Source: CAD feature listing. Evaluate the final solid. Frame: model axes, mm. A direction names the side the tool comes from. Coordinates: 2 decimals unless noted, no trailing zeros. Loops run counter-clockwise (first coordinate to the right, second up) from the corner with the lowest first, then second, coordinate; pieces in that order, holes last. Notation, with made-up numbers: (24.25, 89.25) - (70.25, 89.25) arc R26 cw to (70.25, 104.25) - close; hole circle Ø1 at (-14, -7). An arc over 180 degrees is marked (long way). Use one line per item in the form item = value. Start each with the question number.
from build123d import *

# Parameters (mm, degrees)
SKETCH1_R           = 15.175
SKETCH1_R_2         = 12
BOSS_EXTRUDE1_DEPTH = 20
BOSS_EXTRUDE2_REACH = 57.175
SKETCH2_R           = 12.675
SKETCH2_R_2         = 9.5
SKETCH5_W           = 2.65
SKETCH5_H           = 15.175


with BuildPart() as part:
    # Sketch1 → Boss-Extrude1 (new body, symmetric)
    with BuildSketch(Plane.XY):
        Circle(SKETCH1_R)
        Circle(SKETCH1_R_2, mode=Mode.SUBTRACT)
    extrude(amount=BOSS_EXTRUDE1_DEPTH, both=True)

    # Sketch2 → Boss-Extrude2 (add, up to next)
    with BuildSketch(Plane(origin=(0, 40, 0), x_dir=(1, 0, 0), z_dir=(0, 1, 0)), mode=Mode.PRIVATE) as boss_extrude2_sk1:
        Circle(SKETCH2_R)
        Circle(SKETCH2_R_2, mode=Mode.SUBTRACT)
    boss_extrude2_tool1 = extrude(boss_extrude2_sk1.sketch, amount=-BOSS_EXTRUDE2_REACH, mode=Mode.PRIVATE) - part.part
    add(boss_extrude2_tool1.solids().sort_by_distance((-12.316497, 40, 0))[0])

    # Sketch5 → M5 Clearance Hole1 (revolve, cut)
    with BuildSketch(Plane.ZX.offset(25.5)):
        with Locations((1.325, 7.5875)):
            Rectangle(SKETCH5_W, SKETCH5_H)
    m5_clearance_hole1 = revolve(axis=Axis((-6.35, 25.5, 0), (1, 0, 0)), mode=Mode.SUBTRACT)

    # Mirror1: M5 Clearance Hole1 across plane
    add(m5_clearance_hole1.mirror(Plane(origin=(0, 0, 0), x_dir=(0, 0, 1), z_dir=(1, 0, 0))), mode=Mode.SUBTRACT)


solid = part.part
(1) Mould query, pull axis X, two halves, no side actions, for faces 3 (the face through (-10.923, 23.709, -1.953)), 4 (the face through (12.09, 24.39, -3.81)), 5 (the face through (-11.99, 0.53, -0.28)). Classes: +X half, -X half, draft (parallel to the pull), parting line (faces both ways), or undercut.
(2) Cut plane B-B, the plane z = 0. Output: boundary loops of the cut face in (x, y) (3 decimals).
(3) Contact query for flat-ended pins moving along their axis: pin 1 (2 mm diameter, centred on x = 5, z = -7.5, fed in from -Y); pin 2 (6 mm diameter, centred on y = 27.5, z = 12.5, fed in from -X); pin 3 (1.5 mm diameter, centred on y = 11, z = 9, fed in from +X). Output: stop coordinate, or through.
(4) Cut plane C-C, the plane x = 0. Output: boundary loops of the cut face in (y, z) (3 decimals), plus the area to 3 significant figures.
(5) Material intervals for line 1 (Y direction, x = -10.1, z = 0); line 2 (Y direction, x = 0, z = -10) (3 decimals); line 3 (Y direction, x = 10.35, z = 0), sorted ascending.
(6) Access query for faces 1 (the face through (10, -7, -20)), 2 (the face through (8.776, 26.114, 3.639)). Directions: +Z, -Z, +X, -X, +Y, -Y. A direction counts if a zero-diameter tool reaches every point of the face in a straight line with its end or side. Return the directions, or none.
(7) Cut plane A-A, the plane y = 0. Output: boundary loops of the cut face in (x, z) (3 decimals).
(8) Cut plane D-D, the plane y = 21. Output: boundary loops of the cut face in (x, z) (3 decimals).
Recorded:
q1.face_3 = draft
q1.face_4 = parting line
q1.face_5 = undercut
q2.outline = (-12.675, 8.344) arc R15.175 ccw (long way) to (12.675, 8.344) - (12.675, 22.85) - (9.5, 22.85) - (9.5, 11.833) arc R15.175 ccw to (-9.5, 11.833) - (-9.5, 22.85) - (-12.675, 22.85) - close; (-12.675, 28.15) - (-9.5, 28.15) - (-9.5, 40) - (-12.675, 40) - close; (9.5, 28.15) - (12.675, 28.15) - (12.675, 40) - (9.5, 40) - close; hole circle Ø24 at (0, 0)
q3.pin_1 = -14.64
q3.pin_2 = -8.39
q3.pin_3 = 11.19
q4.outline = (-15.175, -20) - (-12, -20) - (-12, 20) - (-15.175, 20) - close; (12, -20) - (15.175, -20) - (15.175, -12.675) - (40, -12.675) - (40, -9.5) - (15.175, -9.5) - (15.175, 9.5) - (40, 9.5) - (40, 12.675) - (15.175, 12.675) - (15.175, 20) - (12, 20) - close
q4.area = 412 mm²
q5.line_1 = -11.33 to -6.48, 6.48 to 22.85, 28.15 to 40
q5.line_2 = -15.175 to -12, 12 to 40
q5.line_3 = -11.1 to -6.07, 6.07 to 22.85, 28.15 to 40
q6.face_1 = -Z, +X, -X, +Y, -Y
q6.face_2 = +Y
q7.outline = (-15.175, -20) - (-12, -20) - (-12, 20) - (-15.175, 20) - close; (12, -20) - (15.175, -20) - (15.175, 20) - (12, 20) - close
q8.outline = circle Ø25.35 at (0, 0); hole circle Ø19 at (0, 0)
